Input: dimensioned drawing with shaded views. Units: mm. Origin: part minimum x, y, z. A direction names the side the tool comes from. Give positions to 0.01 mm unless a question says otherwise; leave off trailing zeros. Order: outer loops, then holes, each group sorted by start corner. A loop starts at its lowest first (then second) coordinate and runs counter-clockwise, first axis right, second up.
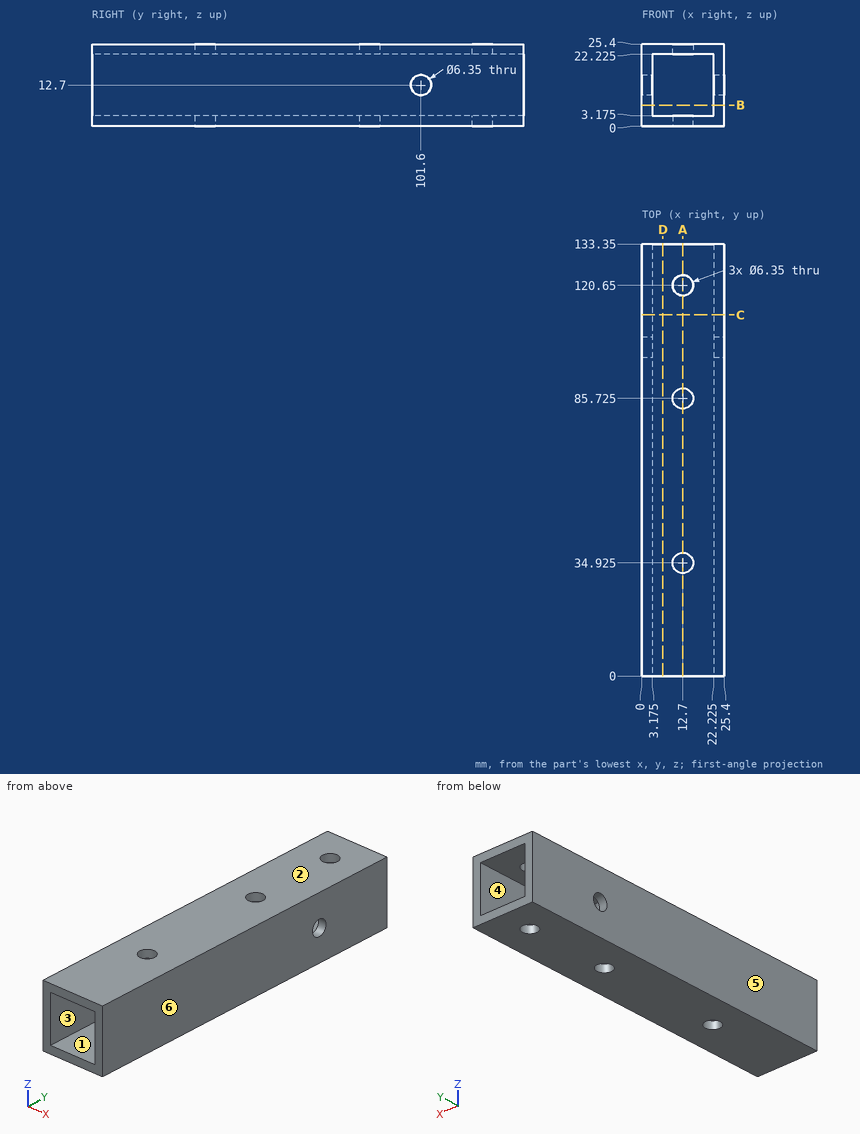
1) Reachability of the marked faces 1 and 2 from +Z, -Z, +X, -X, +Y, -Y: full face, straight path, thin tool, end or side. Return the list, or none.
Report:
face 1: +Y, -Y
face 2: +Z, +X, -X, +Y, -Y
2) Pin query (flat end, axial travel): pin 1 (2 mm diameter, centred on x = 7, y = 56, fed in from -Z); pin 2 (5 mm diameter, centred on x = 12.7, y = 85.725, fed in from -Z). Return the tip coordinate at first contact, or that it passes through.
Report:
pin 1: stops at z = 0
pin 2: passes through
3) Section query C-C, the plane y = 111.5. Return the cut outline in (x, z) (3 decimals).
Report:
outline: (0, 0) - (25.4, 0) - (25.4, 25.4) - (0, 25.4) - close; hole (3.175, 3.175) - (22.225, 3.175) - (22.225, 22.225) - (3.175, 22.225) - close
4) Draft query along X for the marked faces 3, 4, 5 and 6. Return one class per face: +X half, -X half, draft (parallel to the pull), parting line (faces both ways), or undercut.
Report:
face 3: undercut
face 4: undercut
face 5: -X half
face 6: +X half
5) Section query D-D, the plane x = 6.5. Return the cut outline in (y, z) (3 decimals), and give its area (3 significant figures).
Report:
outline: (0, 0) - (133.35, 0) - (133.35, 3.175) - (0, 3.175) - close; (0, 22.225) - (133.35, 22.225) - (133.35, 25.4) - (0, 25.4) - close
area: 847 mm2
6) Section query A-A, the plane x = 12.7. Count the separate pieces of the cut face and the enclosed holes in it, and give its area (3 significant figures).
Report:
separate pieces: 8
enclosed holes: 0
area: 726 mm2
7) Material intervals for L1, parallel to Y at x = 12.7, z = 24.2 (3 decimals); L2, parallel to X at y = 126.5, z = 14.75 (3 decimals), sorted ascending.
Report:
L1: y = 0 to 31.75, 38.1 to 82.55, 88.9 to 117.475, 123.825 to 133.35
L2: x = 0 to 3.175, 22.225 to 25.4
8) Section query B-B, the plane z = 6.5. Return the cut outline in (x, y) (3 decimals), and give its area (3 significant figures).
Report:
outline: (0, 0) - (3.175, 0) - (3.175, 133.35) - (0, 133.35) - close; (22.225, 0) - (25.4, 0) - (25.4, 133.35) - (22.225, 133.35) - close
area: 847 mm2
